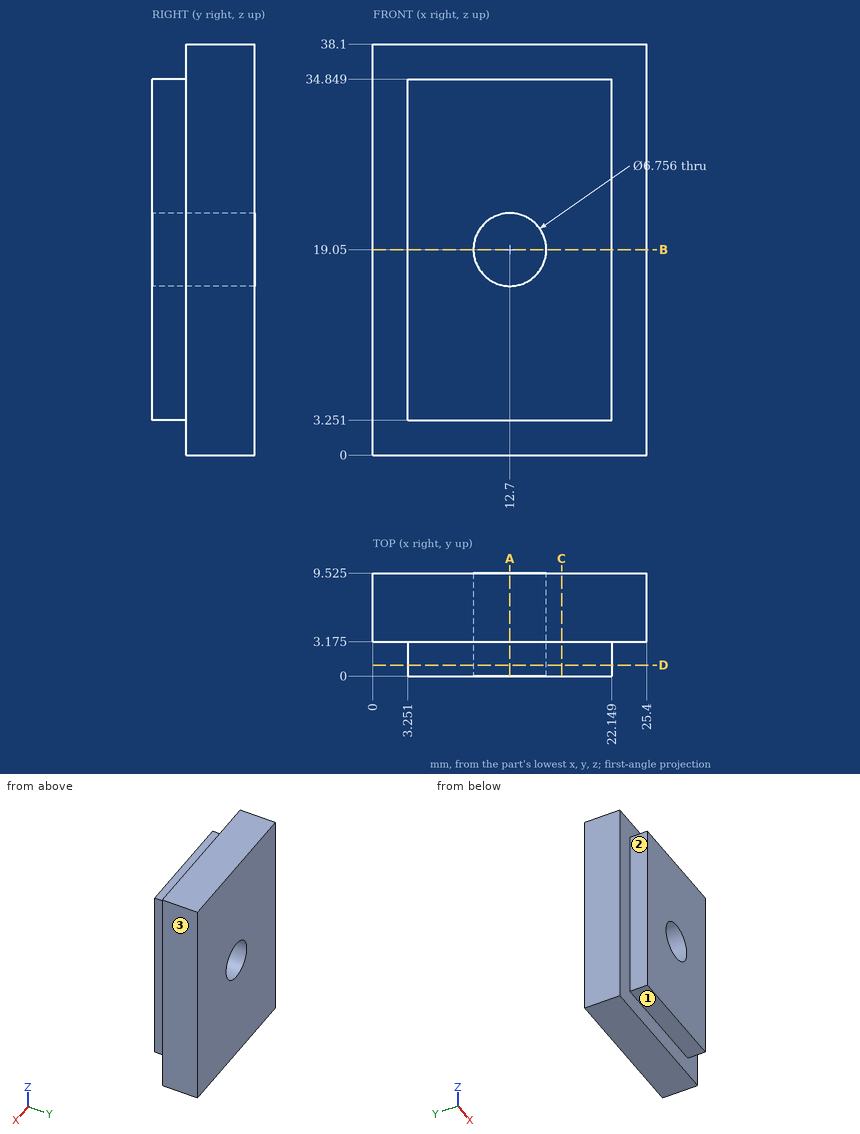
Verification items for this drawing (mm, ordinates from the low corner). A direction names the side the tool comes from. Coordinates: 2 decimals unless noted, no trailing zeros. Write each loop counter-clockwise with the first axis right and the second up, starting at its lowest first coordinate (ties: lowest second). Pieces come first, ordered by that corner, then holes. Notation, with made-up numbers: M 68.5,7.5 L 95.5,7.5 A18 cw 95.5,34.5 Z; hole C 89,10 d10. An arc over 180 degrees is marked long. Answer as a JSON object with one key per item and string values. Group by question number.
(1) Material ranges on line 1 (Z direction, x = 12.7, y = 4); line 2 (Z direction, x = 12.7, y = 3); line 3 (Y direction, x = 2, z = 31.5) (1 decimal), recorded low to high.
(2) Cross-section at D-D, the plane y = 1. Record the cut outline in (x, z).
(3) Gauge pin test, flat ends, axial feed: pin 1 (2.5 mm diameter, centred on x = 9, y = 1.5, fed in from +Z); pin 2 (3.5 mm diameter, centred on y = 1, z = 27, fed in from +X); pin 3 (3.5 mm diameter, centred on x = 11, y = 1, fed in from -Z). Record the tip position at first contact, or that the pin passes through.
(4) Cross-section at B-B, the plane z = 19.05. Record the cut outline in (x, y) (1 decimal), and give its area (3 significant figures).
(5) Cross-section at C-C, the plane x = 17.5. Record the cut outline in (y, z) (1 decimal), and give its area (3 significant figures).
(6) Cross-section at A-A, the plane x = 12.7. Record the cut outline in (y, z) (1 decimal), and give its area (3 significant figures).
(7) Tool access check on the marked faces 1, 2 and 3. Record the directions out of +Z, -Z, +X, -X, +Y, -Y that give a thin tool (end or side, any length) a straight path to the whole face; none if there is none.
Reply:
{
 "1": {"line 1": "0 to 15.67, 22.43 to 38.1", "line 2": "3.25 to 15.67, 22.43 to 34.85", "line 3": "3.2 to 9.5"},
 "2": {"outline": "M 3.25,3.25 L 22.15,3.25 L 22.15,34.85 L 3.25,34.85 Z; hole C 12.7,19.05 d6.76"},
 "3": {"pin 1": "z = 34.85", "pin 2": "x = 22.15", "pin 3": "z = 3.25"},
 "4": {"outline": "M 0,3.2 L 3.3,3.2 L 3.3,0 L 9.3,0 L 9.3,9.5 L 0,9.5 Z; M 16.1,0 L 22.1,0 L 22.1,3.2 L 25.4,3.2 L 25.4,9.5 L 16.1,9.5 Z", "area": "157 mm²"},
 "5": {"outline": "M 0,3.3 L 3.2,3.3 L 3.2,0 L 9.5,0 L 9.5,38.1 L 3.2,38.1 L 3.2,34.8 L 0,34.8 Z", "area": "342 mm²"},
 "6": {"outline": "M 0,3.3 L 3.2,3.3 L 3.2,0 L 9.5,0 L 9.5,15.7 L 0,15.7 Z; M 0,22.4 L 9.5,22.4 L 9.5,38.1 L 3.2,38.1 L 3.2,34.8 L 0,34.8 Z", "area": "278 mm²"},
 "7": {"face 1": "-Z, +X, -X, -Y", "face 2": "+Z, -Z, -X, -Y", "face 3": "+Z, -Z, +X, +Y, -Y"}
}
